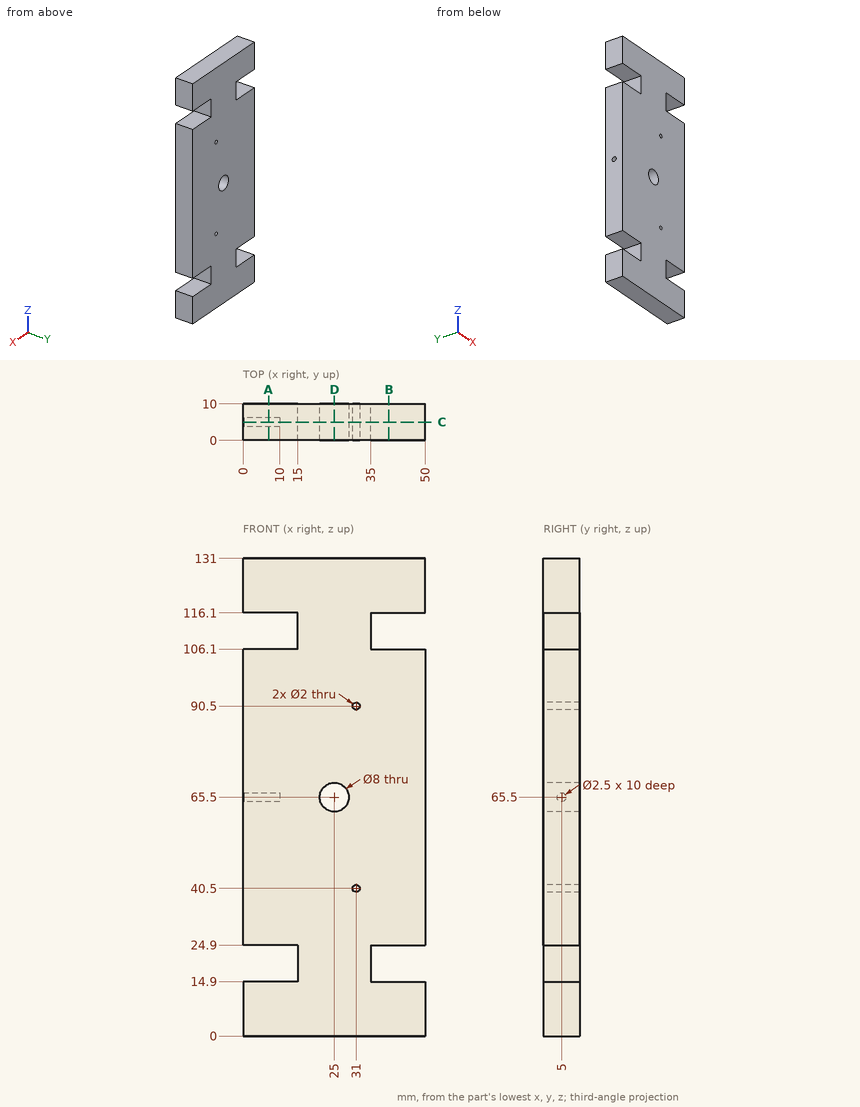
Verification items for this drawing (mm, ordinates from the low corner). Coordinates: 2 decimals unless noted, no trailing zeros. Loops run counter-clockwise (first coordinate to the right, second up) from the corner with the lowest first, then second, coordinate; pieces in that order, holes last. Notation, with made-up numbers: (-19.5, 3) - (10.5, 3) arc R24 cw to (10.5, 31) - close; hole circle Ø6 at (-36.5, 52.25). An arc over 180 degrees is marked (long way). One line per item, written item: value. Start each with the question number.
(1) Cross-section at B-B on x = 40. Enter the section's corners in (y, z).
(2) Material ranges on line 1 (Z direction, x = 31, y = 5.75); line 2 (Z direction, x = 9.5, y = 5.25); line 3 (Z direction, x = 6, y = 2), recorded low to high. Write a range as [from, to].
(3) Cross-section at D-D on x = 25. Enter the section's corners in (y, z).
(4) Depth check by flat-ended pin: P1, Ø3, axis at y = 7, z = 111, coming from the -X side; P2, Ø1.2, axis at y = 5, z = 65.5, coming from the -X side; P3, Ø3, axis at y = 5.5, z = 21.5, coming from the +X side. Enter the tip coordinate at first touch or a pass-through.
(5) Cross-section at A-A on x = 7. Enter the section's corners in (y, z).
(6) Cross-section at C-C on y = 5. Enter the section's corners in (x, z).
Results below:
1. outline: (0, 0) - (10, 0) - (10, 14.9) - (0, 14.9) - close; (0, 24.9) - (10, 24.9) - (10, 106.1) - (0, 106.1) - close; (0, 116.1) - (10, 116.1) - (10, 131) - (0, 131) - close
2. line 1: z = [0, 39.5], [41.5, 89.5], [91.5, 131]
2. line 2: z = [0, 14.9], [24.9, 64.28], [66.72, 106.1], [116.1, 131]
2. line 3: z = [0, 14.9], [24.9, 106.1], [116.1, 131]
3. outline: (0, 0) - (10, 0) - (10, 61.5) - (0, 61.5) - close; (0, 69.5) - (10, 69.5) - (10, 131) - (0, 131) - close
4. P1: stops at x = 15
4. P2: stops at x = 10
4. P3: stops at x = 35
5. outline: (0, 0) - (10, 0) - (10, 14.9) - (0, 14.9) - close; (0, 24.9) - (10, 24.9) - (10, 106.1) - (0, 106.1) - close; (0, 116.1) - (10, 116.1) - (10, 131) - (0, 131) - close; hole circle Ø2.5 at (5, 65.5)
6. outline: (0, 0) - (50, 0) - (50, 14.9) - (35, 14.9) - (35, 24.9) - (50, 24.9) - (50, 106.1) - (35, 106.1) - (35, 116.1) - (50, 116.1) - (50, 131) - (0, 131) - (0, 116.1) - (15, 116.1) - (15, 106.1) - (0, 106.1) - (0, 66.75) - (10, 66.75) - (10, 64.25) - (0, 64.25) - (0, 24.9) - (15, 24.9) - (15, 14.9) - (0, 14.9) - close; hole circle Ø8 at (25, 65.5); hole circle Ø2 at (31, 40.5); hole circle Ø2 at (31, 90.5)
